Design review of the part built by this model. Coordinates are the model's own, in mm. A direction names the side the tool comes from. Coordinates: 2 decimals unless noted, no trailing zeros. Order: outer loops, then holes, each group sorted by start corner. A loop starts at its lowest first (then second) coordinate and runs counter-clockwise, first axis right, second up. Notation, with made-up numbers: (49, 41) -> (101, 41) arc R29 ccw to (101, 80) -> close; hole circle Ø6 at (-32, 87.5). An arc over 180 degrees is marked (long way). Write item = value, one per line.
```python
from build123d import *

# Parameters (mm, degrees)
SKETCH1_W           = 22
SKETCH1_H           = 12
BOSS_EXTRUDE1_DEPTH = 7
CHAMFER1_SIZE       = 2


with BuildPart() as part:
    # Sketch1 → Boss-Extrude1 (new body)
    with BuildSketch(Plane(origin=(0, 0, 0), x_dir=(1, 0, 0), z_dir=(0, 1, 0))):
        with BuildLine():
            Line((26.811555509, 22.502433661), (5.940065191, 49.578823596))
            ThreePointArc((5.940065191, 49.578823596), (-1.362951292, 52.375117882), (-7.184208043, 47.153405394))
            Line((-7.184208043, 47.153405394), (-17, 14.405882918))
            Line((-17, 14.405882918), (-17, -8.881815114))
            ThreePointArc((-17, -8.881815114), (15.805244301, -9.244301568), (43.281511036, 8.682500053))
            Line((43.281511036, 8.682500053), (26.811555509, 22.502433661))
        make_face()
        Rectangle(SKETCH1_W, SKETCH1_H, mode=Mode.SUBTRACT)
    extrude(amount=BOSS_EXTRUDE1_DEPTH)

    # Chamfer1
    chamfer1_edges = [part.edges().sort_by_distance(p)[0] for p in [
        (0, 7, -6),
        (11, 7, 0),
        (0, 7, 6),
        (-11, 7, 0),
    ]]
    chamfer(chamfer1_edges, length=CHAMFER1_SIZE)


solid = part.part
```
(1) We need section B-B (z = 5). Write out the cut boundary in (x, y).
Report:
outline = (-17, 0) -> (-11, 0) -> (-11, 5) -> (-13, 7) -> (-17, 7) -> close; (11, 0) -> (26.31, 0) -> (26.31, 7) -> (13, 7) -> (11, 5) -> close
(2) The part is to be moulded in two halves that separate along Z. For faces 1 (the flat face through (35.162, 3.451, -15.496)), 2 (the flat face through (0, 2, 6)), 3 (the flat face through (6, 0, -14)), say which applies: released by +Z, released by -Z, zero draft, split by the parting line, or undercut.
Report:
face_1 = released by -Z
face_2 = undercut
face_3 = zero draft
(3) We need section A-A (y = 1). Write out the cut boundary in (x, z), and give its area (3 significant figures).
Report:
outline = (-17, -14.41) -> (-7.18, -47.15) arc R7.5 ccw to (5.94, -49.58) -> (26.81, -22.5) -> (43.28, -8.68) arc R56.5 ccw to (-17, 8.88) -> close; hole (-11, -6) -> (11, -6) -> (11, 6) -> (-11, 6) -> close
area = 2,130 mm²
(4) For L1, parallel to Z at x = -5.5, y = 6.5; L2, parallel to Z at x = -3.5, y = 3.5; L3, parallel to X at y = 6, z = 0, list the stretches that pass through material, from the lowest coordinate up.
Report:
L1 = -50.1 to -7.5, 7.5 to 11.23
L2 = -51.63 to -6, 6 to 11.39
L3 = -17 to -12, 12 to 34.17
(5) For faces 4 (the cylindrical face through (-1.25, 3.451, -52.395)), 5 (the flat face through (-12, 6, 0)), 6 (the flat face through (0, 2, -6)), list the 3-axis set-ups (+Z, -Z, +X, -X, +Y, -Y) from which the entire face can be reached by the end or side of a thin tool; tool diameter is ignored.
Report:
face_4 = -Z, +Y, -Y
face_5 = +Y
face_6 = +Y, -Y
(6) We need section C-C (x = -2). Write out the cut boundary in (y, z).
Report:
outline = (0, -52.23) -> (7, -52.23) -> (7, -8) -> (5, -6) -> (0, -6) -> close; (0, 6) -> (5, 6) -> (7, 8) -> (7, 11.46) -> (0, 11.46) -> close
(7) We need section D-D (y = 6). Write out the cut boundary in (x, z).
Report:
outline = (-17, -14.41) -> (-7.18, -47.15) arc R7.5 ccw to (5.94, -49.58) -> (26.81, -22.5) -> (43.28, -8.68) arc R56.5 ccw to (-17, 8.88) -> close; hole (-12, -7) -> (12, -7) -> (12, 7) -> (-12, 7) -> close
(8) Insertion check: pin 1 (3 mm diameter, centred on y = 5.5, z = -11.5, fed in from +X); pin 2 (2.5 mm diameter, centred on y = 1.5, z = 0, fed in from +X); pin 3 (1 mm diameter, centred on y = 5.5, z = -36.5, fed in from -X). Each pin has a flat end and moves straight along its axis. Give the tip position at first contact, or say it passes through.
Report:
pin_1 = 41.71
pin_2 = 35.75
pin_3 = -10.53
